Study the drawing (mm; zero at the part's minimum x, y, z) and answer. A direction names the side the tool comes from. Round coordinates to 2 decimals unless told otherwise and drop trailing zeros. Write each loop counter-clockwise with the first axis right and the second up, starting at its lowest first coordinate (ties: lowest second). Pieces come first, ordered by that corner, then holes. Notation, with made-up numbers: (-36.75, -34.75) - (-15.75, -34.75) arc R32 ccw to (-15.75, -6.75) - close; hole circle Ø7 at (-24, 64.25). An arc over 180 degrees is marked (long way). Return JSON: item names as keys, results as strings. Group by question number.
(1) Which of the six approach directions +Z, -Z, +X, -X, +Y, -Y give full straight-line access (tool end or side, diameter ignored) to the marked faces 4, 5 and 6?
(2) Each of these flat-tipped pins is pushed along its axis until it touches: pin 1 (4.5 mm diameter, centred on x = 16, z = 20, fed in from +Y); pin 2 (5 mm diameter, centred on x = 12.5, y = 9.5, fed in from +Z); pin 3 (2.5 mm diameter, centred on x = 20, y = 22.5, fed in from +Z). Where does it stop, or does it pass through?
(3) Section C-C, the plane z = 22.5 is taken. Write down the section's boundary in (x, y), then the cut area to 3 significant figures.
(4) Determine the mould class of the marked faces 1, 2 and 3 for opening direction X: +X half, -X half, draft (parallel to the pull), parting line (faces both ways), or undercut.
(5) Section D-D, the plane y = 27 is taken. Write down the section's boundary in (x, z).
(6) Section A-A, the plane y = 22.5 is taken. Write down the section's boundary in (x, z).
(7) Section B-B, the plane x = 9.5 is taken. Write down the section's boundary in (y, z).
(8) Find the intervals of material crossed by line 1 along X through (y, z) = (14.5, 10); line 2 along X through (y, z) = (22.5, 11.5); line 3 along Y through (x, z) = (20, 11.2), in increasing order. Write a range as [from, to].
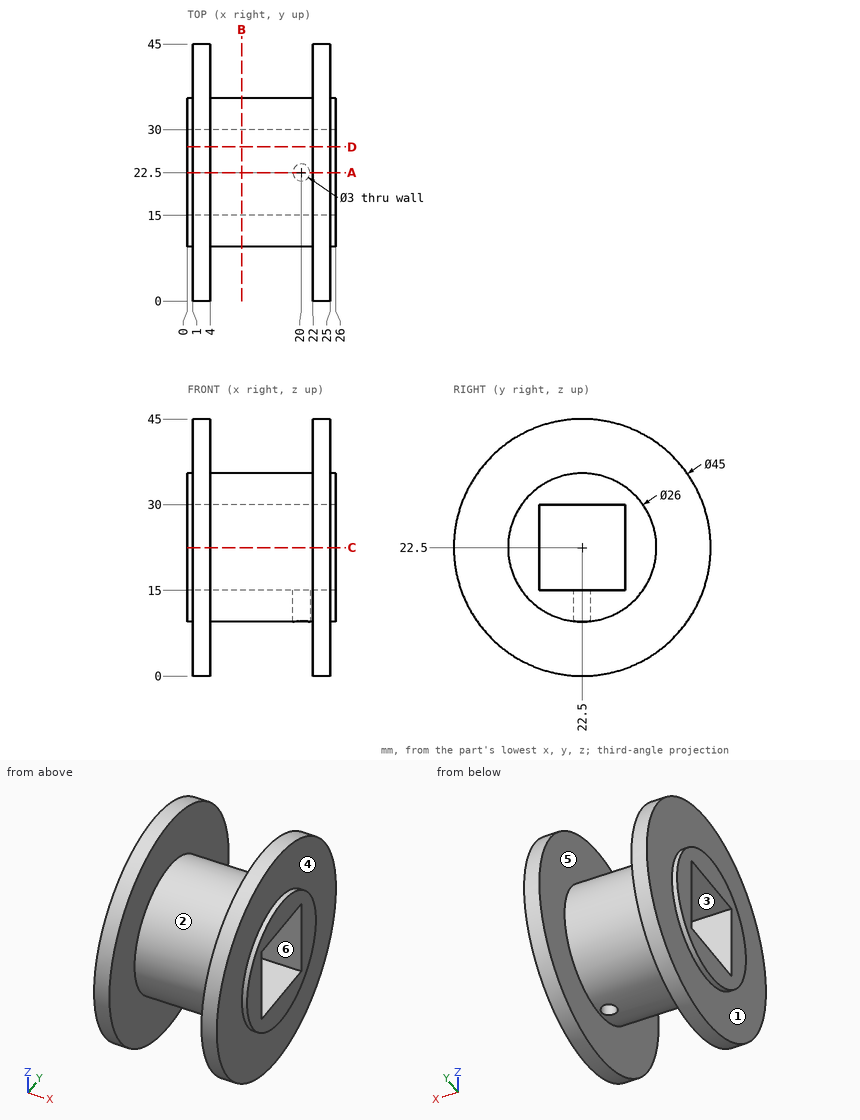
Working result:
{
 "1": {"face 4": "+X", "face 5": "none", "face 6": "+X, -X"},
 "2": {"pin 1": "stops at y = 35.5", "pin 2": "stops at z = 30.16", "pin 3": "stops at z = 35.5"},
 "3": {"outline": "(0, 9.5) - (1, 9.5) - (1, 0) - (4, 0) - (4, 9.5) - (22, 9.5) - (22, 0) - (25, 0) - (25, 9.5) - (26, 9.5) - (26, 15) - (0, 15) - close; (0, 30) - (26, 30) - (26, 35.5) - (25, 35.5) - (25, 45) - (22, 45) - (22, 35.5) - (4, 35.5) - (4, 45) - (1, 45) - (1, 35.5) - (0, 35.5) - close", "area": "400 mm^2"},
 "4": {"face 1": "-X half", "face 2": "undercut", "face 3": "draft"},
 "5": {"outline": "(0, 10.3) - (1, 10.3) - (1, 0.45) - (4, 0.45) - (4, 10.3) - (22, 10.3) - (22, 0.45) - (25, 0.45) - (25, 10.3) - (26, 10.3) - (26, 15) - (0, 15) - close; (0, 30) - (26, 30) - (26, 34.7) - (25, 34.7) - (25, 44.55) - (22, 44.55) - (22, 34.7) - (4, 34.7) - (4, 44.55) - (1, 44.55) - (1, 34.7) - (0, 34.7) - close"},
 "6": {"outline": "(0, 9.5) - (1, 9.5) - (1, 0) - (4, 0) - (4, 9.5) - (18.5, 9.5) - (18.5, 15) - (0, 15) - close; (0, 30) - (26, 30) - (26, 35.5) - (25, 35.5) - (25, 45) - (22, 45) - (22, 35.5) - (4, 35.5) - (4, 45) - (1, 45) - (1, 35.5) - (0, 35.5) - close; (21.5, 9.5) - (22, 9.5) - (22, 0) - (25, 0) - (25, 9.5) - (26, 9.5) - (26, 15) - (21.5, 15) - close"},
 "7": {"outline": "circle Ø26 at (22.5, 22.5); hole (15, 15) - (30, 15) - (30, 30) - (15, 30) - close"},
 "8": {"line 1": "x = [1, 4], [22, 25]", "line 2": "x = [0, 18.5], [21.5, 26]", "line 3": "y = [16.07, 21], [24, 28.93]"}
}
